For this review, take the finished solid that the model builds, in its own axes (mm). A direction names the side the tool comes from. Coordinates: 2 decimals unless noted, no trailing zeros. Write each loop counter-clockwise with the first axis right and the second up, starting at its lowest first coordinate (ties: lowest second). Pieces come first, ordered by that corner, then holes. Notation, with made-up numbers: M 1.25,8 L 38.25,8 A27 ccw 38.25,28 Z; hole C -24,64 d5. An arc over 180 degrees is marked long. One line per question, with ' | ' between items.
from build123d import *

# Parameters (mm, degrees)
F0_W      = 228.6
F0_H      = 38.1
F9_DEPTH  = 6.35
F1_W      = 38.1
F1_H      = 38.1
F1_W_2    = 25.4
F1_H_2    = 25.4
F10_DEPTH = 63.5
F11_W     = 177.8
F11_H     = 38.1
F2_DEPTH  = 6.35
F3_R      = 9.525
F3_R_2    = 3.175
F4_DEPTH  = 25.4
F6_DEPTH  = 6.351
F7_R      = 15.875
F8_DEPTH  = 25.4


with BuildPart() as f9:
    # F0 (on Top) → F9 (new body)
    with BuildSketch(Plane.XY):
        Rectangle(F0_W, F0_H)
    extrude(amount=F9_DEPTH)

    # F1 (on face) → F10 (join)
    with BuildSketch(Plane.XY.offset(6.35)):
        with Locations((69.85, 0)):
            Rectangle(F1_W, F1_H)
        with Locations((69.85, 0)):
            Rectangle(F1_W_2, F1_H_2, mode=Mode.SUBTRACT)
        with Locations((-69.85, 0)):
            Rectangle(F1_W, F1_H)
        with Locations((-69.85, 0)):
            Rectangle(F1_W_2, F1_H_2, mode=Mode.SUBTRACT)
    extrude(amount=F10_DEPTH)

    # F11 (on face) → F2 (join)
    with BuildSketch(Plane.XY.offset(69.85)):
        Rectangle(F11_W, F11_H)
    extrude(amount=F2_DEPTH)

    # F3 (on face) → F4 (cut)
    with BuildSketch(Plane.XY.offset(76.2)):
        Circle(F3_R)
        with Locations((25.4, 0)):
            Circle(F3_R_2)
        with Locations((-25.4, 0)):
            Circle(F3_R_2)
    extrude(amount=-F4_DEPTH, mode=Mode.SUBTRACT)

    # F5 (on face) → F6 (cut, through all)
    with BuildSketch(Plane.XY.offset(6.35)):
        with BuildLine():
            Line((-95.25, 3.175), (-107.95, 3.175))
            ThreePointArc((-107.95, 3.175), (-111.125, 0), (-107.95, -3.175))
            Line((-107.95, -3.175), (-95.25, -3.175))
            ThreePointArc((-95.25, -3.175), (-92.075, 0), (-95.25, 3.175))
        make_face()
        with BuildLine():
            Line((95.25, -3.175), (107.95, -3.175))
            ThreePointArc((107.95, -3.175), (111.125, 0), (107.95, 3.175))
            Line((107.95, 3.175), (95.25, 3.175))
            ThreePointArc((95.25, 3.175), (92.075, 0), (95.25, -3.175))
        make_face()
    extrude(amount=-F6_DEPTH, mode=Mode.SUBTRACT)

    # F7 (on face) → F8 (cut)
    with BuildSketch(Plane(origin=(0, 0, 0), x_dir=(1, 0, 0), z_dir=(0, 0, -1))):
        Circle(F7_R)
    extrude(amount=-F8_DEPTH, mode=Mode.SUBTRACT)


solid = f9.part
1. For line 1 along X through (y, z) = (0, 3) (3 decimals); line 2 along X through (y, z) = (11.5, 53); line 3 along Y through (x, z) = (25.4, 74.25) (3 decimals), list the stretches that pass through material, from the lowest coordinate up.
Computed values:
line 1: x = -114.3 to -111.125, -92.075 to -15.875, 15.875 to 92.075, 111.125 to 114.3 | line 2: x = -88.9 to -82.55, -57.15 to -50.8, 50.8 to 57.15, 82.55 to 88.9 | line 3: y = -19.05 to -3.175, 3.175 to 19.05
2. Take a section at A-A on z = 22.5. State the section outline as (x, y) points.
Computed values:
outline: M -88.9,-19.05 L -50.8,-19.05 L -50.8,19.05 L -88.9,19.05 Z; M 50.8,-19.05 L 88.9,-19.05 L 88.9,19.05 L 50.8,19.05 Z; hole M -82.55,-12.7 L -57.15,-12.7 L -57.15,12.7 L -82.55,12.7 Z; hole M 57.15,-12.7 L 82.55,-12.7 L 82.55,12.7 L 57.15,12.7 Z
3. Take a section at C-C on x = 0. State the section outline as (y, z) points (3 decimals), plus the area to 3 significant figures.
Computed values:
outline: M -19.05,0 L -15.875,0 L -15.875,6.35 L -19.05,6.35 Z; M -19.05,69.85 L -9.525,69.85 L -9.525,76.2 L -19.05,76.2 Z; M 9.525,69.85 L 19.05,69.85 L 19.05,76.2 L 9.525,76.2 Z; M 15.875,0 L 19.05,0 L 19.05,6.35 L 15.875,6.35 Z | area: 161 mm2
4. Take a section at B-B on x = 25.4. State the section outline as (y, z) points (3 decimals).
Computed values:
outline: M -19.05,0 L 19.05,0 L 19.05,6.35 L -19.05,6.35 Z; M -19.05,69.85 L -3.175,69.85 L -3.175,76.2 L -19.05,76.2 Z; M 3.175,69.85 L 19.05,69.85 L 19.05,76.2 L 3.175,76.2 Z
5. Clearance check with flat-ended pins moving along their axes: P1, Ø7.5, axis at x = 99.5, y = -2, coming from the +Z side; P2, Ø1.5, axis at x = 4, y = 6.5, coming from the +Z side; P3, Ø4, axis at y = -15, z = 17.5, coming from the -X side; P4, Ø1, axis at y = 7, z = 63.5, coming from the +X side. State where each tip first meets the part, or that it passes through.
Computed values:
P1: stops at z = 6.35 | P2: passes through | P3: stops at x = -88.9 | P4: stops at x = 88.9
6. Take a section at D-D on x = 67. State the section outline as (y, z) points.
Computed values:
outline: M -19.05,0 L 19.05,0 L 19.05,76.2 L -19.05,76.2 Z; hole M -12.7,6.35 L 12.7,6.35 L 12.7,69.85 L -12.7,69.85 Z
7. Machinability: for faces 4 (the flat face through (102, 3.175, 3)), 5 (the flat face through (70, 0, 6.35)), 6 (the flat face through (-88.9, 0, 41)), 7 (the cylindrical face through (-22.37, 0.95, 73.07)), which of the approach directions +Z, -Z, +X, -X, +Y, -Y give a long, thin tool a straight path to every point of the face, cutting with its end or side? Answer none if there is none.
Computed values:
face 4: +Z, -Z | face 5: none | face 6: +Z, -X, +Y, -Y | face 7: +Z
8. Draft analysis for pull direction Y (two halves, no side actions). For faces 1 (the flat face through (-2, 19.05, 4)), 2 (the flat face through (-50.8, 0, 38)), 3 (the cylindrical face through (28.43, 0.95, 73.07)), state which applies: pulls with the +Y half, pulls with the -Y half, needs draft (parallel to the pull), parting line crosses it, or undercut.
Computed values:
face 1: pulls with the +Y half | face 2: needs draft | face 3: undercut
